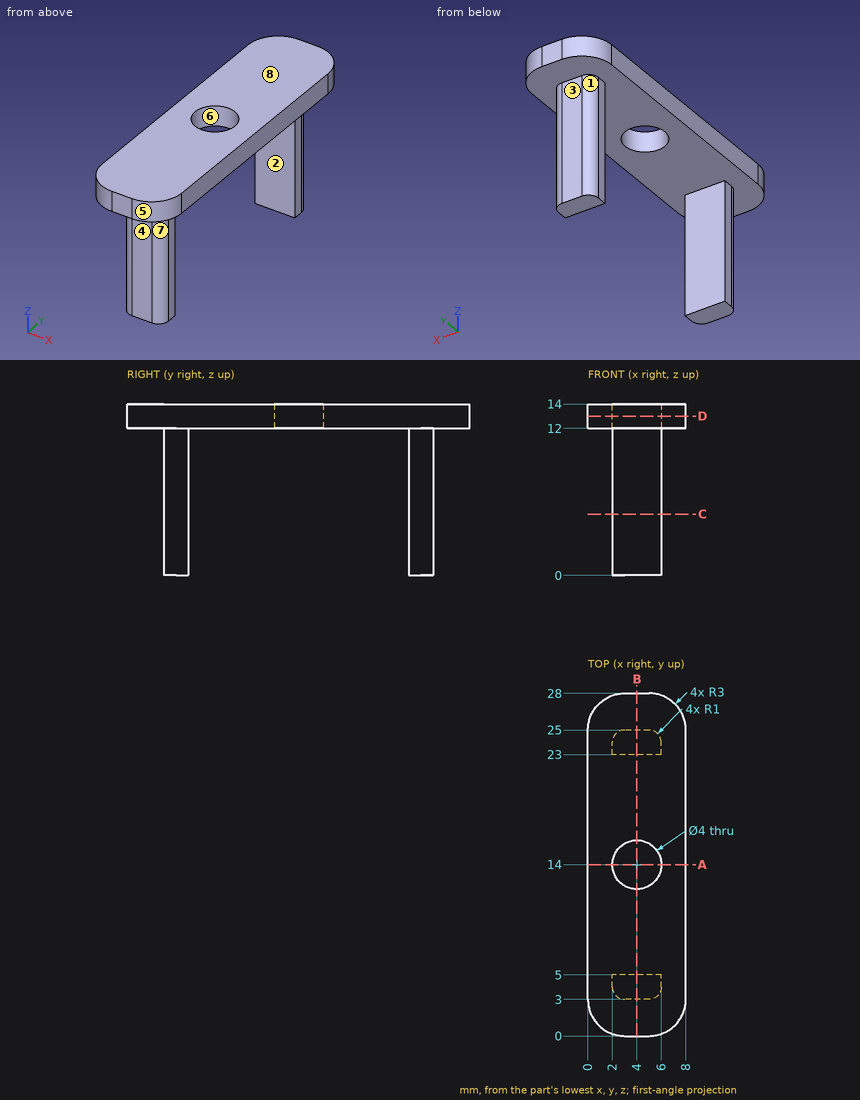
Design review of the part shown in the three views and the two pictorial views. Dimensions are in mm from the part's minimum x, y and z. A direction names the side the tool comes from. Give positions to 0.01 mm unless a question says otherwise; leave off trailing zeros. Loops run counter-clockwise (first coordinate to the right, second up) from the corner with the lowest first, then second, coordinate; pieces in that order, holes last. Notation, with made-up numbers: M -33,10.25 L 23,10.25 A15 ccw 23,30.25 Z; hole C 65,11.25 d3. An arc over 180 degrees is marked long. Answer as a JSON object with one key per item and string values.
Item 1: We need section D-D (z = 13). State the section outline as (x, y) points, and give its area (3 significant figures).
Output values:
{"outline": "M 0,3 A3 ccw 3,0 L 5,0 A3 ccw 8,3 L 8,25 A3 ccw 5,28 L 3,28 A3 ccw 0,25 Z; hole C 4,14 d4", "area": "204 mm2"}
Item 2: Wall thickness on line 1 along Y through (x, z) = (4, 13.3); line 2 along Z through (x, y) = (5.25, 16.5); line 3 along Y through (x, z) = (3.5, 11.25): over which ranges is each line inside the solid? List them lowest first.
Output values:
{"line 1": "y = 0 to 12, 16 to 28", "line 2": "z = 12 to 14", "line 3": "y = 3 to 5, 23 to 25"}
Item 3: Machinability: for the marked faces 1, 2, 3, 4 and 5, which of the approach directions +Z, -Z, +X, -X, +Y, -Y give a long, thin tool a straight path to every point of the face, cutting with its end or side? Answer none if there is none.
Output values:
{"face 1": "-Z, -X, +Y", "face 2": "-Z, +X, -X", "face 3": "-Z, +X, -X, +Y", "face 4": "-Z, +X, -X, -Y", "face 5": "+Z, -Z, +X, -Y"}
Item 4: We need section B-B (x = 4). State the section outline as (y, z) points.
Output values:
{"outline": "M 0,12 L 3,12 L 3,0 L 5,0 L 5,12 L 12,12 L 12,14 L 0,14 Z; M 16,12 L 23,12 L 23,0 L 25,0 L 25,12 L 28,12 L 28,14 L 16,14 Z"}
Item 5: We need section A-A (y = 14). State the section outline as (x, z) points.
Output values:
{"outline": "M 0,12 L 2,12 L 2,14 L 0,14 Z; M 6,12 L 8,12 L 8,14 L 6,14 Z"}
Item 6: We need section C-C (z = 5). State the section outline as (x, y) points.
Output values:
{"outline": "M 2,4 A1 ccw 3,3 L 5,3 A1 ccw 6,4 L 6,5 L 2,5 Z; M 2,23 L 6,23 L 6,24 A1 ccw 5,25 L 3,25 A1 ccw 2,24 Z"}
Item 7: Mouldability with a two-part tool opening along X and no side actions: class the marked faces 6, 7 and 8 as pulls with the +X half, pulls with the -X half, needs draft (parallel to the pull), parting line crosses it, or undercut.
Output values:
{"face 6": "undercut", "face 7": "pulls with the +X half", "face 8": "needs draft"}
Item 8: For P1, Ø3, axis at x = 4.5, z = 4.5, coming from the +Y side; P2, Ø2, axis at y = 25, z = 6, coming from the -X side; P3, Ø0.5, axis at y = 4.5, z = 5.5, coming from the +X side; P4, Ø2.5, axis at x = 4, y = 14, coming from the +Z side (3 decimals), all flat-tipped, find the tip position at first contact; note any pin that passes through.
Output values:
{"P1": "stops at y = 25", "P2": "stops at x = 2", "P3": "stops at x = 6", "P4": "passes through"}
